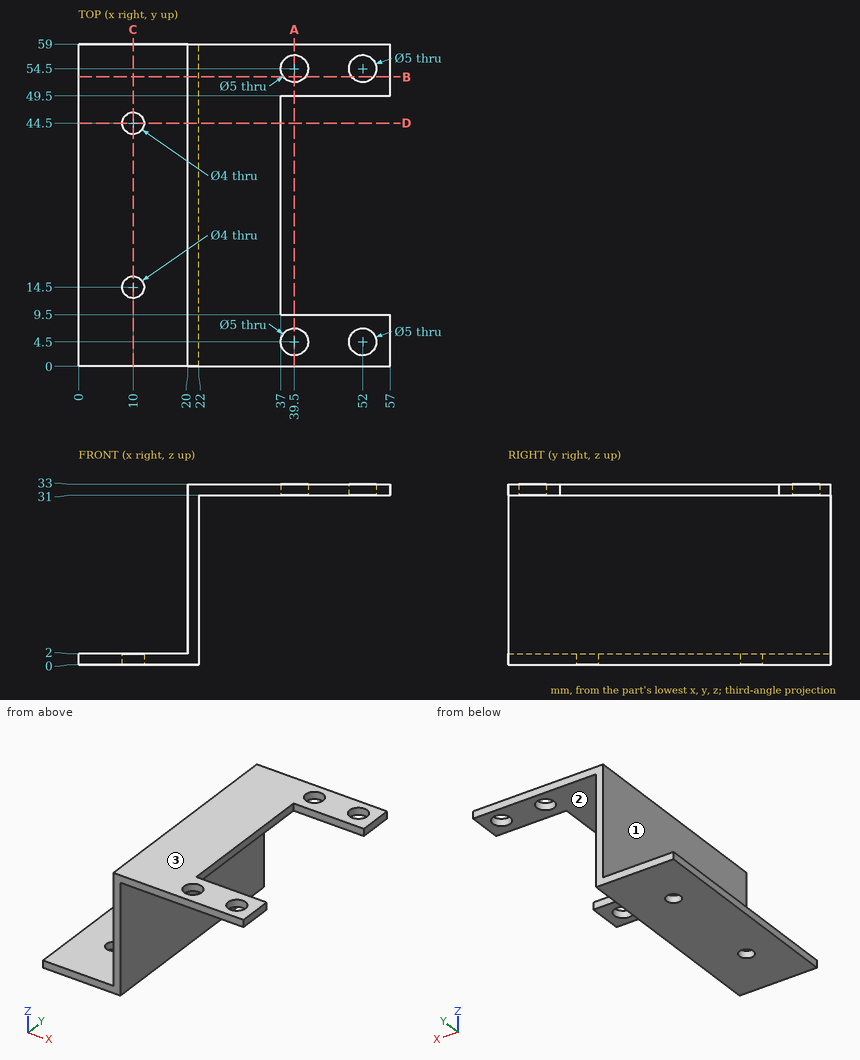
Study the drawing (mm; zero at the part's minimum x, y, z) and answer. A direction names the side the tool comes from. Give positions to 0.01 mm unless a question says otherwise; leave off trailing zeros. Loops run counter-clockwise (first coordinate to the right, second up) from the corner with the lowest first, then second, coordinate; pieces in that order, holes last. Notation, with made-up numbers: (50.25, 26.25) -> (73.25, 26.25) arc R11 ccw to (73.25, 44.25) -> close; hole circle Ø3 at (25.5, -4). An arc over 180 degrees is marked (long way). Use a Markdown table: item, result. Add a question column.
1) The part is cut by section D-D, the plane y = 44.5. Determine the outline of the cut face in (x, z), plus the area to 3 significant figures.
2) The part is cut by section B-B, the plane y = 53. Determine the outline of the cut face in (x, z), plus the area to 3 significant figures.
3) The part is cut by section C-C, the plane x = 10. Determine the outline of the cut face in (y, z).
4) Which of the six approach directions +Z, -Z, +X, -X, +Y, -Y give full straight-line access (tool end or side, diameter ignored) to the marked faces 1, 2 and 3?
5) The part is cut by section A-A, the plane x = 39.5. Determine the outline of the cut face in (y, z), plus the area to 3 significant figures.
6) Consider line 1 along Y through (x, z) = (52, 31.5); line 2 along Y through (x, z) = (10, 0.95); line 3 along Z through (x, y) = (6, 20). Determine where each line is inside the solid, lowest interval first.
7) Each of these flat-tipped pins is pushed along its axis until it touches: P1, Ø2, axis at y = 30.5, z = 32.5, coming from the +X side; P2, Ø1.5, axis at x = 15, y = 51.5, coming from the +Z side; P3, Ø3, axis at y = 33, z = 19.5, coming from the +X side; P4, Ø3, axis at x = 24, z = 6, coming from the +Y side. Where does it stop, or does it pass through?
Reported:
| question | item | result |
|---|---|---|
| 1 | outline | (0, 0) -> (8, 0) -> (8, 2) -> (0, 2) -> close; (12, 0) -> (22, 0) -> (22, 31) -> (37, 31) -> (37, 33) -> (20, 33) -> (20, 2) -> (12, 2) -> close |
| 1 | area | 128 mm^2 |
| 2 | outline | (0, 0) -> (22, 0) -> (22, 31) -> (37.5, 31) -> (37.5, 33) -> (20, 33) -> (20, 2) -> (0, 2) -> close; (41.5, 31) -> (50, 31) -> (50, 33) -> (41.5, 33) -> close; (54, 31) -> (57, 31) -> (57, 33) -> (54, 33) -> close |
| 2 | area | 160 mm^2 |
| 3 | outline | (0, 0) -> (12.5, 0) -> (12.5, 2) -> (0, 2) -> close; (16.5, 0) -> (42.5, 0) -> (42.5, 2) -> (16.5, 2) -> close; (46.5, 0) -> (59, 0) -> (59, 2) -> (46.5, 2) -> close |
| 4 | face 1 | +Z, -X, +Y, -Y |
| 4 | face 2 | -Z, +X, +Y, -Y |
| 4 | face 3 | +Z, +X, -X, +Y, -Y |
| 5 | outline | (0, 31) -> (2, 31) -> (2, 33) -> (0, 33) -> close; (7, 31) -> (9.5, 31) -> (9.5, 33) -> (7, 33) -> close; (49.5, 31) -> (52, 31) -> (52, 33) -> (49.5, 33) -> close; (57, 31) -> (59, 31) -> (59, 33) -> (57, 33) -> close |
| 5 | area | 18.0 mm^2 |
| 6 | line 1 | y = 0 to 2, 7 to 9.5, 49.5 to 52, 57 to 59 |
| 6 | line 2 | y = 0 to 12.5, 16.5 to 42.5, 46.5 to 59 |
| 6 | line 3 | z = 0 to 2 |
| 7 | P1 | stops at x = 37 |
| 7 | P2 | stops at z = 2 |
| 7 | P3 | stops at x = 22 |
| 7 | P4 | passes through |
